from build123d import *

# Parameters (mm, degrees)
BOSS_EXTRUDE1_DEPTH = 1
CUT_EXTRUDE1_REACH  = 46.596
SKETCH2_W           = 30
SKETCH2_H           = 12.5
CUT_EXTRUDE2_REACH  = 46.596
SKETCH3_R           = 2.5


with BuildPart() as part:
    # Sketch1 → Boss-Extrude1 (new, symmetric)
    with BuildSketch(Plane(origin=(0, 0, 0), x_dir=(1, 0, 0), z_dir=(0, 1, 0))):
        with BuildLine():
            Line((-39.278701549, 15), (39.278701549, 15))
            ThreePointArc((39.278701549, 15), (41.95, 0), (39.278701549, -15))
            Line((39.278701549, -15), (-39.278701549, -15))
            ThreePointArc((-39.278701549, -15), (-41.95, 0), (-39.278701549, 15))
        make_face()
    extrude(amount=BOSS_EXTRUDE1_DEPTH, both=True)

    # Sketch2 → Cut-Extrude1 (cut, up to next)
    with BuildSketch(Plane(origin=(0, 1, 0), x_dir=(1, 0, 0), z_dir=(0, 1, 0)), mode=Mode.PRIVATE) as cut_extrude1_sk1:
        with Locations((-41.95, 0)):
            Rectangle(SKETCH2_W, SKETCH2_H)
    cut_extrude1_tool1 = extrude(cut_extrude1_sk1.sketch, amount=-CUT_EXTRUDE1_REACH, mode=Mode.PRIVATE) & part.part
    add(cut_extrude1_tool1.solids().sort_by_distance((-41.95, 1, 0))[0], mode=Mode.SUBTRACT)

    # Sketch3 → Cut-Extrude2 (cut, up to next)
    with BuildSketch(Plane.XZ.offset(1), mode=Mode.PRIVATE) as cut_extrude2_sk1:
        with Locations(Location((15.778701549, 8, 0), (0, 0, 270))):
            Circle(SKETCH3_R)
    cut_extrude2_tool1 = extrude(cut_extrude2_sk1.sketch, amount=-CUT_EXTRUDE2_REACH, mode=Mode.PRIVATE) & part.part
    # Sketch3 → Cut-Extrude2 (cut, up to next)
    with BuildSketch(Plane.XZ.offset(1), mode=Mode.PRIVATE) as cut_extrude2_sk2:
        with Locations(Location((15.778701549, -8, 0), (0, 0, 270))):
            Circle(SKETCH3_R)
    cut_extrude2_tool2 = extrude(cut_extrude2_sk2.sketch, amount=-CUT_EXTRUDE2_REACH, mode=Mode.PRIVATE) & part.part
    add(cut_extrude2_tool1.solids().sort_by_distance((15.778702, -1, 8))[0], mode=Mode.SUBTRACT)
    add(cut_extrude2_tool2.solids().sort_by_distance((15.778702, -1, -8))[0], mode=Mode.SUBTRACT)


solid = part.part
Input: part model. Units: mm. Frame: model coordinates. A direction names the side the tool comes from. Round coordinates to 2 decimals unless told otherwise and drop trailing zeros. Write each loop counter-clockwise with the first axis right and the second up, starting at its lowest first coordinate (ties: lowest second). Pieces come first, ordered by that corner, then holes.
1) Cut plane A-A (z = -8). Return the cut outline in (x, y), then the cut area to 3 significant figures.
2) Cut plane B-B (y = 0.6). Return the cut outline in (x, z).
3) Contact query for a flat-ended pin moving along its axis: P1, Ø3, axis at x = 15.78, z = -8, coming from the +Y side. Output: stop coordinate, or through.
4) Cut plane C-C (z = 13). Return the cut outline in (x, y).
5) Draft query along Z for faces 3 (the cylindrical face through (13.56, -0.01, -9.15)), 4 (the flat face through (1, 1, 0)), 5 (the cylindrical face through (41.95, 0.01, -0.21)), 6 (the flat face through (-34, 0, 6.25)). Return one class per face: pulls with the +Z half, pulls with the -Z half, needs draft (parallel to the pull), parting line crosses it, or undercut.
6) Ray query, L1, parallel to Z at x = 16, y = 0.4; L2, parallel to X at y = -0.5, z = -8; L3, parallel to X at y = 0, z = 7. Return the intervals inside material, ascending.
7) Reachability of faces 1 (the flat face through (-34, 0, -6.25)), 2 (the cylindrical face through (13.338, -0.014, 8.542)) from +Z, -Z, +X, -X, +Y, -Y: full face, straight path, thin tool, end or side. Return the list, or none.
Geometry says:
1. outline: (-41.21, -1) - (13.28, -1) - (13.28, 1) - (-41.21, 1) - close; (18.28, -1) - (41.21, -1) - (41.21, 1) - (18.28, 1) - close
1. area: 155 mm2
2. outline: (-41.5, -6.25) arc R43.45 ccw to (-39.28, -15) - (39.28, -15) arc R43.45 ccw to (39.28, 15) - (-39.28, 15) arc R43.45 ccw to (-41.5, 6.25) - (-26.95, 6.25) - (-26.95, -6.25) - close; hole circle Ø5 at (15.78, -8); hole circle Ø5 at (15.78, 8)
3. P1: passes through
4. outline: (-39.96, -1) - (39.96, -1) - (39.96, 1) - (-39.96, 1) - close
5. face 3: undercut
5. face 4: needs draft
5. face 5: parting line crosses it
5. face 6: undercut
6. L1: z = -15 to -10.49, -5.51 to 5.51, 10.49 to 15
6. L2: x = -41.21 to 13.28, 18.28 to 41.21
6. L3: x = -41.38 to 13.49, 18.07 to 41.38
7. face 1: -X, +Y, -Y
7. face 2: +Y, -Y
